The model under review builds one solid part; all positions refer to its coordinate system, in mm. A direction names the side the tool comes from. Round coordinates to 2 decimals unless told otherwise and drop trailing zeros. Write each loop counter-clockwise with the first axis right and the second up, starting at its lowest first coordinate (ties: lowest second). Pieces come first, ordered by that corner, then holes. Notation, with made-up numbers: (73, -29) -> (97, -29) arc R17 cw to (97, -11) -> close; hole circle Ø7 at (-39, -14). An arc over 180 degrees is marked (long way). Return JSON: item names as keys, results as strings. Group by question number.
1. For line 1 along X through (y, z) = (1.05, 22.5); line 2 along X through (y, z) = (2.35, 27); line 3 along X through (y, z) = (2.1, 7), list the stretches that pass through material, from the lowest coordinate up. Write a range as from..to.
2. Take a section at C-C, the plane x = 6.5. Write out the cut boundary in (y, z) (3 decimals).
3. Take a section at A-A, the plane y = 1.7. Give the number of separate pieces and of enclosed holes in the cut face, then the cut area to 3 significant figures.
4. Take a section at B-B, the plane x = 22. Write out the cut boundary in (y, z) (3 decimals), then the cut area to 3 significant figures.
5. Mouldability with a two-part tool opening along Z and no side actions: class faces 3 (the flat face through (1, 0, 2)), 4 (the cylindrical face through (-70.812, 1.61, 12.6)), 5 (the cylindrical face through (-59.09, 1.61, 33.01)), 6 (the cylindrical face through (-58.94, 1.61, 19.19)) as pulls with the +Z half, pulls with the -Z half, needs draft (parallel to the pull), parting line crosses it, or undercut.
6. Tool access review of faces 1 (the flat face through (34.979, 1.565, 20.195)), 2 (the cylindrical face through (59.306, 1.61, 17.122)): name each direction out of +Z, -Z, +X, -X, +Y, -Y from which nothing blocks a thin tool from reaching the whole face with its end or side.
from build123d import *

# Parameters (mm, degrees)
BOSS_EXTRUDE1_DEPTH = 3.175
SKETCH2_R           = 3.4925
CUT_EXTRUDE2_DEPTH  = 3.175
LPATTERN5_COUNT     = 3
LPATTERN5_PITCH     = 22.86
SKETCH7_R           = 3.4925
CUT_EXTRUDE3_DEPTH  = 3.175
LPATTERN6_COUNT     = 3
LPATTERN6_PITCH     = 22.86
FILLET1_R           = 3.175
FILLET3_R           = 3.175
FILLET4_R           = 25.4


with BuildPart() as part:
    # Sketch1 → Boss-Extrude1 (new body)
    with BuildSketch(Plane(origin=(0, 0, 0), x_dir=(1, 0, 0), z_dir=(0, 1, 0))):
        Polygon((-25.4, 14.664696837), (0, 29.329393675), (25.4, 14.664696837), (72.092022192, -12.292954744), (59.392022192, -34.29), (0, 0), (-59.392022192, -34.29), (-72.092022192, -12.292954744), align=None)
    extrude(amount=BOSS_EXTRUDE1_DEPTH)

    # Sketch2 → Cut-Extrude2 (cut)
    with BuildSketch(Plane(origin=(0, 3.175, 0), x_dir=(1, 0, 0), z_dir=(0, 1, 0))):
        with Locations(Location((-55.843351826, -17.576477372, 0), (0, 0, 270))):
            Circle(SKETCH2_R)
    cut_extrude2 = extrude(amount=-CUT_EXTRUDE2_DEPTH, mode=Mode.SUBTRACT)

    # LPattern5: Cut-Extrude2 ×3
    with Locations(*[Vector(0.8660254037844386, 0, -0.5000000000000002) * (i * LPATTERN5_PITCH) for i in range(1, LPATTERN5_COUNT)]):
        add(cut_extrude2, mode=Mode.SUBTRACT)

    # Sketch7 → Cut-Extrude3 (cut)
    with BuildSketch(Plane(origin=(0, 3.175, 0), x_dir=(1, 0, 0), z_dir=(0, 1, 0))):
        with Locations(Location((55.843351826, -17.576477372, 0), (0, 0, 270))):
            Circle(SKETCH7_R)
    cut_extrude3 = extrude(amount=-CUT_EXTRUDE3_DEPTH, mode=Mode.SUBTRACT)

    # LPattern6: Cut-Extrude3 ×3
    with Locations(*[Vector(-0.8660254037844377, 0, -0.5000000000000017) * (i * LPATTERN6_PITCH) for i in range(1, LPATTERN6_COUNT)]):
        add(cut_extrude3, mode=Mode.SUBTRACT)

    # Fillet1
    fillet1_edges = [part.edges().sort_by_distance(p)[0] for p in [
        (72.092022192, 1.5875, 12.292954744),
        (59.392022192, 1.5875, 34.29),
        (-59.392022192, 1.5875, 34.29),
        (-72.092022192, 1.5875, 12.292954744),
    ]]
    fillet(fillet1_edges, radius=FILLET1_R)

    # Fillet3
    fillet3_edges = [part.edges().sort_by_distance(p)[0] for p in [
        (0, 1.5875, -29.329393675),
    ]]
    fillet(fillet3_edges, radius=FILLET3_R)

    # Fillet4
    fillet4_edges = [part.edges().sort_by_distance(p)[0] for p in [
        (0, 1.5875, 0),
    ]]
    fillet(fillet4_edges, radius=FILLET4_R)


solid = part.part
Output:
{
 "1": {"line 1": "x = -66.2..-38.97, 38.97..66.2", "line 2": "x = -63.6..-46.77, 46.77..63.6", "line 3": "x = -62.92..-39.43, -32.66..-12.11, 12.11..32.66, 39.43..62.92"},
 "2": {"outline": "(0, -25.577) -> (3.175, -25.577) -> (3.175, 4.775) -> (0, 4.775) -> close"},
 "3": {"separate pieces": "1", "enclosed holes": "6", "area": "3,650 mm^2"},
 "4": {"outline": "(0, -16.628) -> (3.175, -16.628) -> (3.175, 12.702) -> (0, 12.702) -> close", "area": "93.1 mm^2"},
 "5": {"face 3": "needs draft", "face 4": "parting line crosses it", "face 5": "pulls with the +Z half", "face 6": "undercut"},
 "6": {"face 1": "+Z, +Y, -Y", "face 2": "+Y, -Y"}
}
